Can you work these out from the drawing? Everything is in mm from the part's minimum corner. A direction names the side the tool comes from. Round coordinates to 2 decimals unless told otherwise and drop trailing zeros. Write each loop counter-clockwise with the first axis right and the second up, starting at its lowest first coordinate (ties: lowest second). Pieces come first, ordered by that corner, then holes.
Q1. If we section it at C-C (x = 78.5): Please give me the cut outline in (y, z), plus the area to 4 significant figures.
Q2. Please list where these lines run through material, in increasing order: line 1 along Y through (x, z) = (78, 71.5); line 2 along X through (y, z) = (41, 58.5); line 3 along X through (y, z) = (23.5, 6.5).
Q3. I'm going to push flat-ended pins straight in: pin 1 Ø2 at (x, z) = (64.5, 18) entering from +Y; pin 2 Ø6 at (x, y) = (67.5, 30) entering from +Z. Where does each tip first touch, or does it pass through?
Q4. We'd pull the mould along X, two halves only. Please class the marked faces 4, 5, 6 and 7: +X half, -X half, draft (parallel to the pull), parting line (faces both ways), or undercut.
Q5. If we section it at A-A (y = 60): Please give me the cut outline in (x, z), plus the area to 3 significant figures.
Q6. For the marked faces 1, 2 and 3, which set-ups out of +Z, -Z, +X, -X, +Y, -Y let a thin tool reach every point of the face, with its end or its side?
Q7. If we section it at D-D (z = 69): Please give me the cut outline in (x, y), plus the area to 3 significant figures.
Q8. If we section it at B-B (z = 51.5): Please give me the cut outline in (x, y), plus the area to 3 significant figures.
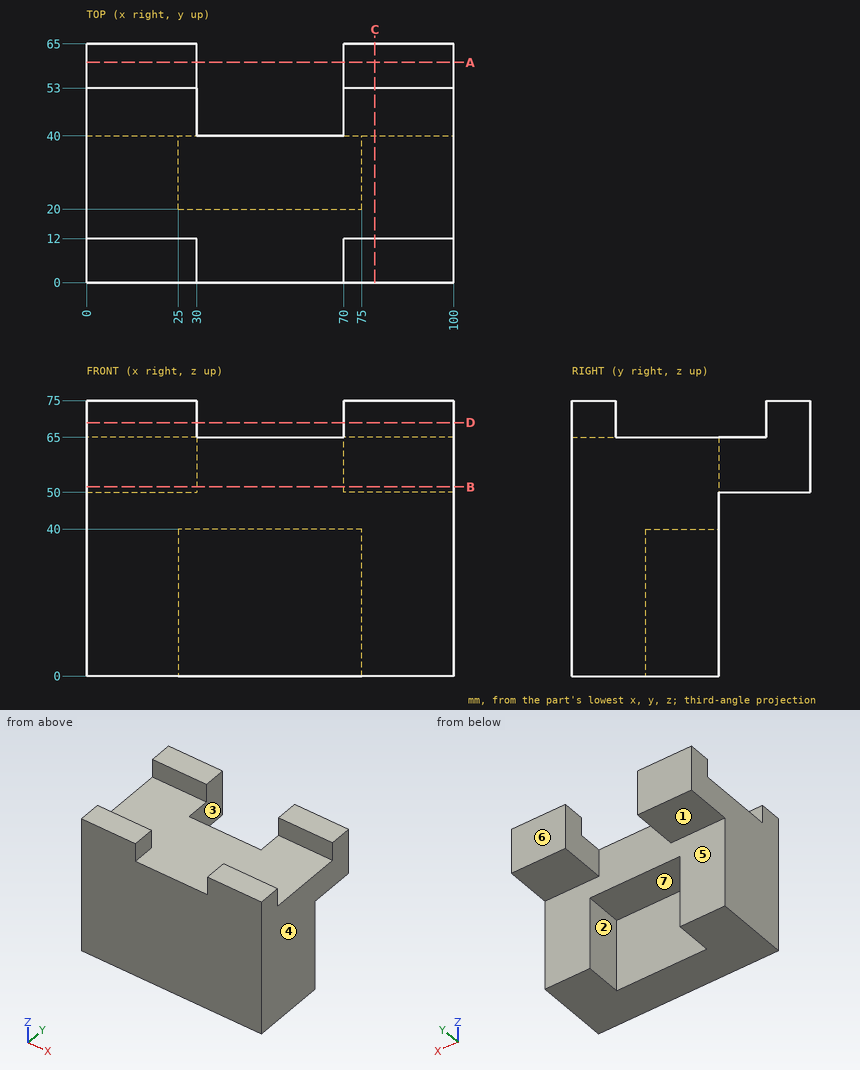
A:
1. outline: (0, 0) - (40, 0) - (40, 50) - (65, 50) - (65, 75) - (53, 75) - (53, 65) - (12, 65) - (12, 75) - (0, 75) - close
1. area: 3,215 mm2
2. line 1: y = 0 to 12, 53 to 65
2. line 2: x = 0 to 30, 70 to 100
2. line 3: x = 0 to 25, 75 to 100
3. pin 1: stops at y = 20
3. pin 2: stops at z = 65
4. face 4: +X half
4. face 5: undercut
4. face 6: draft
4. face 7: undercut
5. outline: (0, 50) - (30, 50) - (30, 75) - (0, 75) - close; (70, 50) - (100, 50) - (100, 75) - (70, 75) - close
5. area: 1,500 mm2
6. face 1: -Z, +X, -X, +Y
6. face 2: -Z, +Y
6. face 3: +Z, -Z, +Y
7. outline: (0, 0) - (30, 0) - (30, 12) - (0, 12) - close; (0, 53) - (30, 53) - (30, 65) - (0, 65) - close; (70, 0) - (100, 0) - (100, 12) - (70, 12) - close; (70, 53) - (100, 53) - (100, 65) - (70, 65) - close
7. area: 1,440 mm2
8. outline: (0, 0) - (100, 0) - (100, 65) - (70, 65) - (70, 40) - (30, 40) - (30, 65) - (0, 65) - close
8. area: 5,500 mm2
